```python
from build123d import *

# Parameters (mm, degrees)
F0_W     = 50.8
F0_H     = 25.4
F1_DEPTH = 38.1
F3_DEPTH = 12.7


# Not quite as in the source:
# - a length typed as a fraction of an inch, garbled in the dataset ("3 / 203.2 mm" for 3/8 in), is restored


with BuildPart() as f1:
    # F0 (on Front) → F1 (new body)
    with BuildSketch(Plane.XZ):
        with Locations((25.4, 12.7)):
            Rectangle(F0_W, F0_H)
    extrude(amount=F1_DEPTH)

    # F2 (on face) → F3 (cut)
    with BuildSketch(Plane.XY.offset(25.4)):
        Polygon((31.75, 0), (6.35, -38.1), (44.45, -38.1), (50.8, -19.05), (50.8, 0), align=None)
    extrude(amount=-F3_DEPTH, mode=Mode.SUBTRACT)


solid = f1.part
```
Model file for the job. Use its own axes, mm. A direction names the side the tool comes from. Give positions to 0.01 mm unless a question says otherwise; leave off trailing zeros. Write each loop counter-clockwise with the first axis right and the second up, starting at its lowest first coordinate (ties: lowest second). Pieces come first, ordered by that corner, then holes. Notation, with made-up numbers: (2, -14) -> (15, -14) arc R31 cw to (15, 20) -> close; hole circle Ø4 at (-25.75, -37). An arc over 180 degrees is marked (long way). Use CSV: the item, a comma, the result in double quotes. Start each with the question number.
1) Cut at C-C on x = 33. List the corners of the cut face in (y, z).
2) Cut at B-B on y = -21. List the corners of the cut face in (x, z), plus the area to 3 significant figures.
3) Pin check, flat tips, straight feed: P1, Ø6, axis at x = 11, z = 22, coming from the -Y side (3 decimals); P2, Ø6, axis at x = 38, y = -9.5, coming from the -Z side; P3, Ø8, axis at x = 35, y = -13, coming from the +Z side; P4, Ø5, axis at x = 19.5, z = 18.5, coming from the -Y side (3 decimals). Stop position of each tip, or through.
4) Cut at A-A on z = 16.25. List the corners of the cut face in (x, y), plus the area to 3 significant figures.
5) Cut at D-D on y = -3. List the corners of the cut face in (x, z).
6) Tool access for faces 1 (the flat face through (47.58, -28.71, 19.14)), 2 (the flat face through (19.23, -18.78, 19.14)), 3 (the flat face through (33, -19, 12.7)): list every direction of +Z, -Z, +X, -X, +Y, -Y with a clear straight run to the whole face (end or side of a thin tool).
7) Drill centre lines: L1, parallel to Z at x = 28.5, y = -8; L2, parallel to Y at x = 18.5, z = 17 (3 decimals); L3, parallel to Y at x = 29, z = 14.75 (3 decimals). Where is each one in solid material? Low to high.
Final values:
1,outline,"(-38.1, 0) -> (0, 0) -> (0, 12.7) -> (-38.1, 12.7) -> close"
2,outline,"(0, 0) -> (50.8, 0) -> (50.8, 25.4) -> (50.15, 25.4) -> (50.15, 12.7) -> (17.75, 12.7) -> (17.75, 25.4) -> (0, 25.4) -> close"
2,area,"879 mm2"
3,P1,"stops at y = -35.625"
3,P2,"stops at z = 0"
3,P3,"stops at z = 12.7"
3,P4,"stops at y = -22.125"
4,outline,"(0, -38.1) -> (6.35, -38.1) -> (31.75, 0) -> (0, 0) -> close; (44.45, -38.1) -> (50.8, -38.1) -> (50.8, -19.05) -> close"
4,area,"786 mm2"
5,outline,"(0, 0) -> (50.8, 0) -> (50.8, 12.7) -> (29.75, 12.7) -> (29.75, 25.4) -> (0, 25.4) -> close"
6,face 1,"+Z, +Y"
6,face 2,"+Z, -Y"
6,face 3,"+Z"
7,L1,"z = 0 to 12.7"
7,L2,"y = -19.875 to 0"
7,L3,"y = -4.125 to 0"
